Read the model definition and answer for the solid it produces. Units are mm, in the model's axes. A direction names the side the tool comes from. Coordinates: 2 decimals unless noted, no trailing zeros. Loops run counter-clockwise (first coordinate to the right, second up) from the corner with the lowest first, then second, coordinate; pieces in that order, holes last.
from build123d import *

# Parameters (mm, degrees)
SKETCH1_R           = 1.5
SKETCH1_R_2         = 3.96875
BOSS_EXTRUDE1_DEPTH = 1.5875
FILLET1_R           = 1.5875


with BuildPart() as part:
    # Sketch1 → Boss-Extrude1 (new, symmetric)
    # profile 1 of 3: a face of its own
    with BuildSketch(Plane(origin=(0, 0, 0), x_dir=(1, 0, 0), z_dir=(0, 1, 0))):
        with BuildLine():
            Line((-2.232421875, 11.695087928), (-38.99296875, 4.678035171))
            ThreePointArc((-38.99296875, 4.678035171), (-42.8625, 0), (-38.99296875, -4.678035171))
            Line((-38.99296875, -4.678035171), (-2.232421875, -11.695087928))
            ThreePointArc((-2.232421875, -11.695087928), (-0.48273715, -11.896459722), (1.277510766, -11.837514744))
            Line((1.277510766, -11.837514744), (88.9, -2.38125))
            ThreePointArc((88.9, -2.38125), (87.216201977, -1.683798023), (86.51875, 0))
            Line((86.51875, 0), (86.51875, 6.35))
            ThreePointArc((86.51875, 6.35), (77.7875, 1.528980536), (69.05625, 6.35))
            Line((69.05625, 6.35), (69.05625, 0))
            ThreePointArc((69.05625, 0), (66.675, -2.38125), (64.29375, 0))
            Line((64.29375, 0), (64.29375, 6.35))
            ThreePointArc((64.29375, 6.35), (64.991201977, 8.033798023), (66.675, 8.73125))
            Line((66.675, 8.73125), (0.568744164, 11.892658203))
            ThreePointArc((0.568744164, 11.892658203), (-0.837683941, 11.876745121), (-2.232421875, 11.695087928))
        make_face()
        with Locations(Location((-38.1, 0, 0), (0, 0, 270))):
            Circle(SKETCH1_R, mode=Mode.SUBTRACT)
        with Locations(Location((0, 0, 0), (0, 0, 270))):
            Circle(SKETCH1_R_2, mode=Mode.SUBTRACT)
    # profile 2 of 3: a face of its own
    with BuildSketch(Plane(origin=(0, 0, 0), x_dir=(1, 0, 0), z_dir=(0, 1, 0))):
        with BuildLine():
            ThreePointArc((69.05625, 6.35), (68.358798023, 8.033798023), (66.675, 8.73125))
            ThreePointArc((66.675, 8.73125), (64.991201977, 8.033798023), (64.29375, 6.35))
            Line((64.29375, 6.35), (64.29375, 0))
            ThreePointArc((64.29375, 0), (66.675, -2.38125), (69.05625, 0))
            Line((69.05625, 0), (69.05625, 6.35))
        make_face()
    # profile 3 of 3: a face of its own
    with BuildSketch(Plane(origin=(0, 0, 0), x_dir=(1, 0, 0), z_dir=(0, 1, 0))):
        with BuildLine():
            ThreePointArc((86.51875, 0), (87.216201977, -1.683798023), (88.9, -2.38125))
            ThreePointArc((88.9, -2.38125), (90.583798023, -1.683798023), (91.28125, 0))
            Line((91.28125, 0), (91.28125, 6.35))
            ThreePointArc((91.28125, 6.35), (88.9, 8.73125), (86.51875, 6.35))
            Line((86.51875, 6.35), (86.51875, 0))
        make_face()
    extrude(amount=BOSS_EXTRUDE1_DEPTH, both=True)

    # Fillet1
    fillet1_edges = [part.edges().sort_by_distance(p)[0] for p in [
        (69.05625, 0, -6.35),
        (86.51875, 0, -6.35),
    ]]
    fillet(fillet1_edges, radius=FILLET1_R)


solid = part.part
Q1. Determine the mould class of faces 1 (the face through (-3.874, -0.022, -0.86)), 2 (the face through (-0.507, 0.022, 11.895)), 3 (the face through (-20.355, 0.022, -8.236)) for opening direction Z: +Z half, -Z half, draft (parallel to the pull), parting line (faces both ways), or undercut.
Findings below:
face 1: undercut
face 2: +Z half
face 3: -Z half
Q2. A cutting plane is placed at B-B (z = 6.25). Give the vertices of the cut face in (x, y).
Findings below:
outline: (-30.76, -1.59) - (53.05, -1.59) - (53.05, 1.59) - (-30.76, 1.59) - close
Q3. A cutting plane is placed at A-A (y = -1.1). Count the separate pieces of the cut face and the enclosed holes in it, then the cut area to 3 significant figures.
Findings below:
separate pieces: 1
enclosed holes: 2
area: 2,070 mm2
Q4. A cutting plane is placed at C-C (x = 36.5). Give the vertices of the cut face in (y, z).
Findings below:
outline: (-1.59, -10.17) - (1.59, -10.17) - (1.59, 8.04) - (-1.59, 8.04) - close
Q5. Straight lines are drawn through the part: probe 1 along X at (y, z) = (0.1, -2.75); probe 2 along Z at (x, y) = (39.5, 1.4); probe 3 along Z at (x, y) = (11, 0.3). For each, find the intervals that lie inside material, in ascending order.
Findings below:
probe 1: x = -41.99 to -2.86, 2.86 to 72.92, 82.66 to 91.28
probe 2: z = -10.03 to 7.71
probe 3: z = -11.39 to 10.79
Q6. Which of the six approach directions +Z, -Z, +X, -X, +Y, -Y give full straight-line access (tool end or side, diameter ignored) to faces 4 (the face through (23, 1.588, 0)), 5 (the face through (68.26, -0.022, -8.127))?
Findings below:
face 4: +Z, -Z, +X, -X, +Y
face 5: -Z, +Y, -Y
Q7. Flat-ended cylindrical pins translate along their axes: pin 1 Ø1 at (x, y) = (55, -1) entering from -Z; pin 2 Ø1.5 at (x, y) = (1.5, -1) entering from +Z; pin 3 Ø1 at (x, y) = (25.5, -0.5) entering from -Z. Find the tip coordinate at first contact, or state that the pin passes through.
Findings below:
pin 1: stops at z = -9.31
pin 2: stops at z = 11.88
pin 3: stops at z = -10.72
